Check sheet for the modelled part. Datum: model origin and axes. Units: mm. Give positions to 0.01 mm unless a question says otherwise; leave off trailing zeros. Write each loop counter-clockwise with the first axis right and the second up, starting at its lowest first coordinate (ties: lowest second). Pieces come first, ordered by that corner, then holes. Notation, with made-up numbers: M -15,54.5 L -10,54.5 A15 cw -10,73.5 Z; hole C 17,-1.75 d8. An arc over 180 degrees is marked long. Write item = value, one per line. Start each with the question number.
1) Cross-section at B-B, the plane y = -1. Record the cut outline in (x, z), plus the area to 3 significant figures.
2) Scan lines: line 1 along Z through (x, y) = (9, 17.5); line 2 along Z through (x, y) = (-90, 22). Record each from-to range of solid material in increasing order. Write a range as [from, to].
3) Cross-section at A-A, the plane x = -701.5. Record the cut outline in (y, z).
```python
from build123d import *

# Parameters (mm, degrees)
F0_W     = 42
F0_H     = 42
F1_DEPTH = 1400


with BuildPart() as f1:
    # F0 (on Right) → F1 (new body, symmetric)
    with BuildSketch(Plane.YZ):
        with BuildLine():
            Line((21, 25), (-21, 25))
            ThreePointArc((-21, 25), (-23.828427, 23.828427), (-25, 21))
            Line((-25, 21), (-25, -21))
            ThreePointArc((-25, -21), (-23.828427, -23.828427), (-21, -25))
            Line((-21, -25), (21, -25))
            ThreePointArc((21, -25), (23.828427, -23.828427), (25, -21))
            Line((25, -21), (25, 21))
            ThreePointArc((25, 21), (23.828427, 23.828427), (21, 25))
        make_face()
        Rectangle(F0_W, F0_H, mode=Mode.SUBTRACT)
    extrude(amount=F1_DEPTH, both=True)


solid = f1.part
```
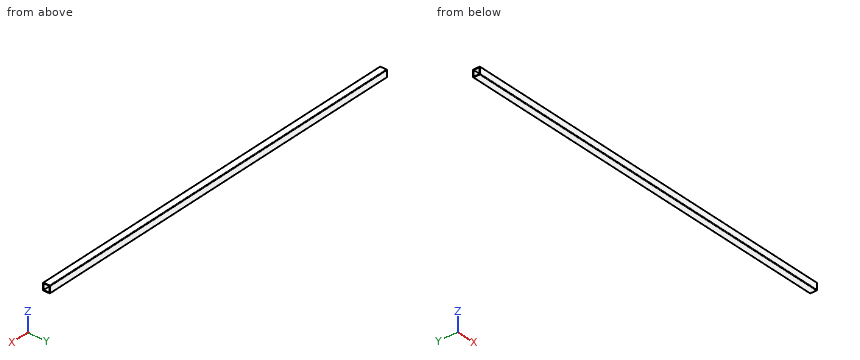
Reply:
q1.outline = M -1400,-25 L 1400,-25 L 1400,-21 L -1400,-21 Z; M -1400,21 L 1400,21 L 1400,25 L -1400,25 Z
q1.area = 22,400 mm2
q2.line_1 = [-25, -21], [21, 25]
q2.line_2 = [-24.87, 24.87]
q3.outline = M -25,-21 A4 ccw -21,-25 L 21,-25 A4 ccw 25,-21 L 25,21 A4 ccw 21,25 L -21,25 A4 ccw -25,21 Z; hole M -21,-21 L 21,-21 L 21,21 L -21,21 Z
